Geometry: final body of the model. Coordinates: model frame, mm. Face numbers are marked on the shaded views. A direction names the side the tool comes from. Give positions to 0.01 mm unless a question says otherwise; leave off trailing zeros. Loops run counter-clockwise (first coordinate to the right, second up) from the corner with the lowest first, then second, coordinate; pieces in that order, holes last. Notation, with made-up numbers: (17.25, 29.5) -> (71.25, 29.5) arc R18 ccw to (71.25, 45.5) -> close; hole circle Ø2 at (87.5, 80). An arc over 180 degrees is marked (long way). Answer in a Markdown table with one row per item. Add a question column.
1) Section query C-C (y = 10). Return the cut outline in (x, z), plus the area to 3 significant figures.
2) Access query for the marked faces 3 and 4. Directions: +Z, -Z, +X, -X, +Y, -Y. A direction counts if a zero-diameter tool reaches every point of the face in a straight line with its end or side. Return the directions, or none.
3) First-contact query: P1, Ø0.6, axis at x = -2, y = 0, coming from the +Z side; P2, Ø1, axis at y = 5, z = 7, coming from the +X side; P3, Ø4, axis at x = 5, z = 3.5, coming from the -Y side. Flat tips, straight axial feed; report the tip coordinate or a pass-through.
4) Draft query along Y for the marked faces 1 and 2. Return one class per face: +Y half, -Y half, draft (parallel to the pull), parting line (faces both ways), or undercut.
5) Line query: line 1 (X direction, y = -15, z = 10.5); line 2 (X direction, y = -2.5, z = 8.75); line 3 (Z direction, x = -7, y = -1). Output: solid intervals per line, ascending. Write a range as from..to.
6) Section query A-A (x = 0). Return the cut outline in (y, z).
7) Section query B-B (z = 2.75). Give the number of separate pieces and of enclosed holes in the cut face, plus the area to 3 significant figures.
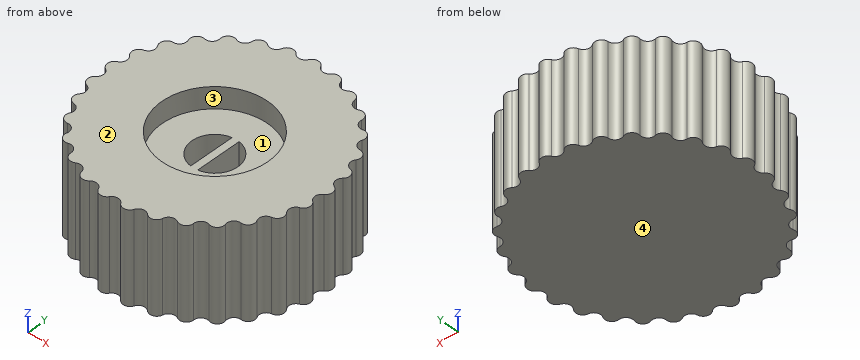
```python
from build123d import *

# Parameters (mm, degrees)
BOSS_EXTRUDE1_DEPTH = 13
SKETCH4_R           = 3.25
CUT_EXTRUDE1_DEPTH  = 12
SKETCH5_R           = 7.5
CUT_EXTRUDE2_DEPTH  = 3
SKETCH6_W           = 1
SKETCH6_H           = 6.908542988
BOSS_EXTRUDE4_DEPTH = 9
FILLET1_R           = 1


with BuildPart() as part:
    # Sketch1 → Boss-Extrude1 (new body)
    with BuildSketch(Plane.XY):
        with BuildLine():
            ThreePointArc((-0.866208619, 15.475777287), (0, 16), (0.866208619, 15.475777287))
            ThreePointArc((0.866208619, 15.475777287), (1.626702908, 14.957286238), (2.480877513, 15.300171462))
            ThreePointArc((2.480877513, 15.300171462), (3.439527043, 15.625928891), (4.172791799, 14.927752966))
            ThreePointArc((4.172791799, 14.927752966), (4.804045905, 14.257900157), (5.71196057, 14.409146625))
            ThreePointArc((5.71196057, 14.409146625), (6.718225625, 14.521206715), (7.284259872, 13.681723507))
            ThreePointArc((7.284259872, 13.681723507), (7.756757055, 12.891830512), (8.675958699, 12.844366106))
            ThreePointArc((8.675958699, 12.844366106), (9.682787443, 12.737489051), (10.055124049, 11.795951863))
            ThreePointArc((10.055124049, 11.795951863), (10.346770866, 10.9229532), (11.234278642, 10.678997303))
            ThreePointArc((11.234278642, 10.678997303), (12.194592882, 10.358180557), (12.355821801, 9.35861462))
            ThreePointArc((12.355821801, 9.35861462), (12.452981171, 8.443330736), (13.267296201, 8.014290456))
            ThreePointArc((13.267296201, 8.014290456), (14.136192711, 7.494535051), (14.078775059, 6.483678959))
            ThreePointArc((14.078775059, 6.483678959), (13.976903916, 5.568907511), (14.679949736, 4.974844294))
            ThreePointArc((14.679949736, 4.974844294), (15.41679988, 4.280453416), (15.143420442, 3.305573676))
            ThreePointArc((15.143420442, 3.305573676), (14.847282169, 2.434088361), (15.406185137, 1.702779942))
            ThreePointArc((15.406185137, 1.702779942), (15.976534622, 0.866222537), (15.499976315, -0.027096558))
            ThreePointArc((15.499976315, -0.027096558), (15.023418009, -0.814546056), (15.412044443, -1.648904508))
            ThreePointArc((15.412044443, -1.648904508), (15.789224361, -2.588511945), (15.131770524, -3.358499787))
            ThreePointArc((15.131770524, -3.358499787), (14.49707552, -4.025093205), (14.697253681, -4.923488015))
            ThreePointArc((14.697253681, -4.923488015), (14.863627517, -5.922210485), (14.05601996, -6.532863299))
            ThreePointArc((14.05601996, -6.532863299), (13.292865893, -7.047431469), (13.295235671, -7.967854695))
            ThreePointArc((13.295235671, -7.967854695), (13.243023971, -8.978993046), (12.323025525, -9.401757384))
            ThreePointArc((12.323025525, -9.401757384), (11.46709663, -9.74023967), (11.271547218, -10.639653345))
            ThreePointArc((11.271547218, -10.639653345), (11.003191342, -11.615927871), (10.013820113, -11.831035743))
            ThreePointArc((10.013820113, -11.831035743), (9.105138673, -11.97760509), (8.720813745, -12.81395363))
            ThreePointArc((8.720813745, -12.81395363), (8.248861715, -13.709714819), (7.236379601, -13.70710802))
            ThreePointArc((7.236379601, -13.70710802), (6.317434552, -13.654911008), (5.762304713, -14.389087685))
            ThreePointArc((5.762304713, -14.389087685), (5.108824482, -15.162450739), (4.120574023, -14.94225116))
            ThreePointArc((4.120574023, -14.94225116), (3.234334213, -14.693728463), (2.534356717, -15.291403992))
            ThreePointArc((2.534356717, -15.291403992), (1.729904295, -15.906207314), (0.812094982, -15.478711243))
            ThreePointArc((0.812094982, -15.478711243), (0, -15.045483507), (-0.812094982, -15.478711243))
            ThreePointArc((-0.812094982, -15.478711243), (-1.729904295, -15.906207314), (-2.534356717, -15.291403992))
            ThreePointArc((-2.534356717, -15.291403992), (-3.234334213, -14.693728463), (-4.120574023, -14.94225116))
            ThreePointArc((-4.120574023, -14.94225116), (-5.108824482, -15.162450739), (-5.762304713, -14.389087685))
            ThreePointArc((-5.762304713, -14.389087685), (-6.317434552, -13.654911008), (-7.236379601, -13.70710802))
            ThreePointArc((-7.236379601, -13.70710802), (-8.248861715, -13.709714819), (-8.720813745, -12.81395363))
            ThreePointArc((-8.720813745, -12.81395363), (-9.105138673, -11.97760509), (-10.013820113, -11.831035743))
            ThreePointArc((-10.013820113, -11.831035743), (-11.003191342, -11.615927871), (-11.271547218, -10.639653345))
            ThreePointArc((-11.271547218, -10.639653345), (-11.46709663, -9.74023967), (-12.323025525, -9.401757384))
            ThreePointArc((-12.323025525, -9.401757384), (-13.243023971, -8.978993046), (-13.295235671, -7.967854695))
            ThreePointArc((-13.295235671, -7.967854695), (-13.292865893, -7.047431469), (-14.05601996, -6.532863299))
            ThreePointArc((-14.05601996, -6.532863299), (-14.863627517, -5.922210485), (-14.697253681, -4.923488015))
            ThreePointArc((-14.697253681, -4.923488015), (-14.49707552, -4.025093205), (-15.131770524, -3.358499787))
            ThreePointArc((-15.131770524, -3.358499787), (-15.789224361, -2.588511945), (-15.412044443, -1.648904508))
            ThreePointArc((-15.412044443, -1.648904508), (-15.023418009, -0.814546056), (-15.499976315, -0.027096558))
            ThreePointArc((-15.499976315, -0.027096558), (-15.976534622, 0.866222537), (-15.406185137, 1.702779942))
            ThreePointArc((-15.406185137, 1.702779942), (-14.847282169, 2.434088361), (-15.143420442, 3.305573676))
            ThreePointArc((-15.143420442, 3.305573676), (-15.41679988, 4.280453416), (-14.679949736, 4.974844294))
            ThreePointArc((-14.679949736, 4.974844294), (-13.976903916, 5.568907511), (-14.078775059, 6.483678959))
            ThreePointArc((-14.078775059, 6.483678959), (-14.136192711, 7.494535051), (-13.267296201, 8.014290456))
            ThreePointArc((-13.267296201, 8.014290456), (-12.452981171, 8.443330736), (-12.355821801, 9.35861462))
            ThreePointArc((-12.355821801, 9.35861462), (-12.194592882, 10.358180557), (-11.234278642, 10.678997303))
            ThreePointArc((-11.234278642, 10.678997303), (-10.346770866, 10.9229532), (-10.055124049, 11.795951863))
            ThreePointArc((-10.055124049, 11.795951863), (-9.682787443, 12.737489051), (-8.675958699, 12.844366106))
            ThreePointArc((-8.675958699, 12.844366106), (-7.756757055, 12.891830512), (-7.284259872, 13.681723507))
            ThreePointArc((-7.284259872, 13.681723507), (-6.718225625, 14.521206715), (-5.71196057, 14.409146625))
            ThreePointArc((-5.71196057, 14.409146625), (-4.804045905, 14.257900157), (-4.172791799, 14.927752966))
            ThreePointArc((-4.172791799, 14.927752966), (-3.439527043, 15.625928891), (-2.480877513, 15.300171462))
            ThreePointArc((-2.480877513, 15.300171462), (-1.626702908, 14.957286238), (-0.866208619, 15.475777287))
        make_face()
    extrude(amount=BOSS_EXTRUDE1_DEPTH)

    # Sketch4 → Cut-Extrude1 (cut)
    with BuildSketch(Plane.XY.offset(13)):
        Circle(SKETCH4_R)
    extrude(amount=-CUT_EXTRUDE1_DEPTH, mode=Mode.SUBTRACT)

    # Sketch5 → Cut-Extrude2 (cut)
    with BuildSketch(Plane.XY.offset(13)):
        Circle(SKETCH5_R)
    extrude(amount=-CUT_EXTRUDE2_DEPTH, mode=Mode.SUBTRACT)

    # Sketch6 → Boss-Extrude4 (add)
    with BuildSketch(Plane.XY.offset(1)):
        Rectangle(SKETCH6_W, SKETCH6_H)
    extrude(amount=BOSS_EXTRUDE4_DEPTH)

    # Fillet1
    fillet1_edges = [part.edges().sort_by_distance(p)[0] for p in [
        (-3.25, 0, 1),
        (3.25, 0, 1),
        (0.5, 0, 1),
        (-0.5, 0, 1),
    ]]
    fillet(fillet1_edges, radius=FILLET1_R)


solid = part.part
```
Evaluation:
| question | item | result |
|---|---|---|
| 1 | outline | (-12.39, 0) -> (12.39, 0) -> (12.39, 13) -> (-12.39, 13) -> close |
| 1 | area | 322 mm² |
| 2 | face 3 | +Z |
| 2 | face 4 | -Z, +X, -X, +Y, -Y |
| 3 | P1 | z = 1 |
| 3 | P2 | x = 15.33 |
| 3 | P3 | y = -15.21 |
| 4 | face 1 | undercut |
| 4 | face 2 | draft |
| 5 | line 1 | -5.41..-4.19, -2.71..2.71, 4.19..5.41 |
| 5 | line 2 | -15.8..-2.08, -0.5..0.5, 2.08..15.8 |
| 5 | line 3 | 0..10 |
| 6 | outline | (-15.05, 0) -> (16, 0) -> (16, 13) -> (7.5, 13) -> (7.5, 10) -> (-7.5, 10) -> (-7.5, 13) -> (-15.05, 13) -> close |
| 7 | separate pieces | 1 |
| 7 | enclosed holes | 2 |
| 7 | area | 731 mm² |
